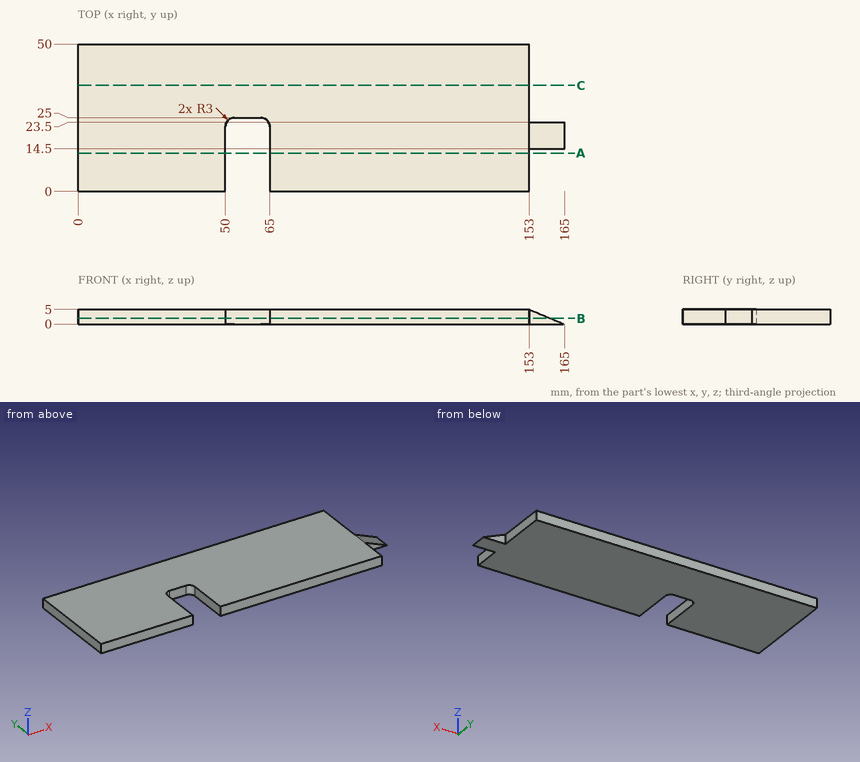
Geometry: see drawing. Coordinates: mm, zero at the bounding-box minimum. Round coordinates to 2 decimals unless told otherwise and drop trailing zeros. Order: outer loops, then holes, each group sorted by start corner. A loop starts at its lowest first (then second) coordinate and runs counter-clockwise, first axis right, second up. Notation, with made-up numbers: (47, 28) - (86, 28) arc R21 ccw to (86, 65) - close; hole circle Ø2 at (45.5, -39.75). An arc over 180 degrees is marked (long way). Use a Markdown table: item, result. Add a question column.
1. Line query: probe 1 along X at (y, z) = (9, 0.95); probe 2 along X at (y, z) = (29.5, 1.6); probe 3 along X at (y, z) = (16, 0.55). Output: solid intervals per line, ascending.
2. First-contact query: pin 1 (1.5 mm diameter, centred on y = 33, z = 1.5, fed in from +X); pin 2 (2.5 mm diameter, centred on x = 159.5, z = 3.5, fed in from -Y); pin 3 (2.5 mm diameter, centred on x = 57, z = 2, fed in from -Y). Flat tips, straight axial feed; report the tip coordinate or a pass-through.
3. Section query C-C (y = 36). Return the cut outline in (x, z), then the cut area to 3 significant figures.
4. Section query B-B (z = 2). Return the cut outline in (x, y).
5. Section query A-A (y = 13). Return the cut outline in (x, z), then the cut area to 3 significant figures.
Derived:
| question | item | result |
|---|---|---|
| 1 | probe 1 | 0 to 50, 65 to 153 |
| 1 | probe 2 | 0 to 153 |
| 1 | probe 3 | 0 to 50, 65 to 163.68 |
| 2 | pin 1 | x = 153 |
| 2 | pin 2 | y = 14.5 |
| 2 | pin 3 | y = 25 |
| 3 | outline | (0, 0) - (153, 0) - (153, 5) - (0, 5) - close |
| 3 | area | 765 mm2 |
| 4 | outline | (0, 0) - (50, 0) - (50, 22) arc R3 cw to (53, 25) - (62, 25) arc R3 cw to (65, 22) - (65, 0) - (153, 0) - (153, 14.5) - (160.2, 14.5) - (160.2, 23.5) - (153, 23.5) - (153, 50) - (0, 50) - close |
| 5 | outline | (0, 0) - (50, 0) - (50, 5) - (0, 5) - close; (65, 0) - (153, 0) - (153, 5) - (65, 5) - close |
| 5 | area | 690 mm2 |
